from build123d import *

# Parameters (mm, degrees)
F0_R     = 1
F0_W     = 8.5
F0_H     = 8
F0_H_2   = 0.5
F1_DEPTH = 1
F2_DEPTH = 3.65
F3_DEPTH = 5.5


with BuildPart() as f1:
    # F0 (on Top) → F1 (new body)
    with BuildSketch(Plane.XY):
        Polygon((12.5, -12), (12.5, 12), (-12.5, 12), (-12.5, -12), (-10.25, -12), (-10.25, -6.25), (-4.25, -6.25), (-4.25, 1.75), (4.25, 1.75), (4.25, -6.25), (10.25, -6.25), (10.25, -12), align=None)
        with Locations((-10.5, -2.5)):
            Circle(F0_R, mode=Mode.SUBTRACT)
        with Locations((10.5, -2.5)):
            Circle(F0_R, mode=Mode.SUBTRACT)
        with Locations((-10.5, 10)):
            Circle(F0_R, mode=Mode.SUBTRACT)
        with Locations((10.5, 10)):
            Circle(F0_R, mode=Mode.SUBTRACT)
        Polygon((-10.25, -12), (10.25, -12), (10.25, -6.25), (4.25, -6.25), (4.25, -6.75), (-4.25, -6.75), (-4.25, -6.25), (-10.25, -6.25), align=None)
        with Locations((0, -2.25)):
            Rectangle(F0_W, F0_H)
        with Locations((0, -6.5)):
            Rectangle(F0_W, F0_H_2)
    extrude(amount=-F1_DEPTH)

    # F0 (on Top) → F2 (join)
    with BuildSketch(Plane.XY):
        Polygon((-10.25, -12), (10.25, -12), (10.25, -6.25), (4.25, -6.25), (4.25, -6.75), (-4.25, -6.75), (-4.25, -6.25), (-10.25, -6.25), align=None)
        with Locations((0, -6.5)):
            Rectangle(F0_W, F0_H_2)
    extrude(amount=-F2_DEPTH)

    # F0 (on Top) → F3 (join)
    with BuildSketch(Plane.XY):
        with Locations((0, -2.25)):
            Rectangle(F0_W, F0_H)
        with Locations((0, -6.5)):
            Rectangle(F0_W, F0_H_2)
    extrude(amount=F3_DEPTH)


solid = f1.part
Verification items for the finished model (mm, model axes). A direction names the side the tool comes from. Coordinates: 2 decimals unless noted, no trailing zeros. Order: outer loops, then holes, each group sorted by start corner. A loop starts at its lowest first (then second) coordinate and runs counter-clockwise, first axis right, second up. Notation, with made-up numbers: M -32.5,-35 L -2.5,-35 A8 cw -2.5,-26 Z; hole C -34,47.25 d3. An arc over 180 degrees is marked long. Write each question's results on one line, items separated by ' | '.
1) Scan lines: line 1 along Y through (x, z) = (10.5, -0.45); line 2 along Y through (x, z) = (9, -2.25); line 3 along Z through (x, y) = (-5, -1.75). Record each from-to range of solid material in increasing order. Write a range as [from, to].
Solved:
line 1: y = [-12, -3.5], [-1.5, 9], [11, 12] | line 2: y = [-12, -6.25] | line 3: z = [-1, 0]
2) Release check for a two-part mould opening along Y. For faces 4 (the face through (9.7, -3.1, -0.5)), 5 (the face through (0, -6.25, -2)), 6 (the face through (0, 3, 0)) record: pulls with the +Y half, pulls with the -Y half, needs draft (parallel to the pull), parting line crosses it, or undercut.
Solved:
face 4: undercut | face 5: pulls with the +Y half | face 6: needs draft
3) Section check D-D on x = 2. Record the cut outline in (y, z).
Solved:
outline: M -12,-3.65 L -6.25,-3.65 L -6.25,-1 L 12,-1 L 12,0 L 1.75,0 L 1.75,5.5 L -6.75,5.5 L -6.75,0 L -12,0 Z
4) Section check A-A on y = 10. Record the cut outline in (x, z), plus the area to 3 significant figures.
Solved:
outline: M -12.5,-1 L -11.5,-1 L -11.5,0 L -12.5,0 Z; M -9.5,-1 L 9.5,-1 L 9.5,0 L -9.5,0 Z; M 11.5,-1 L 12.5,-1 L 12.5,0 L 11.5,0 Z | area: 21.0 mm²
5) Gauge pin test, flat ends, axial feed: pin 1 Ø2 at (x, y) = (5.5, -2) entering from -Z; pin 2 Ø3 at (x, z) = (0, 3) entering from -Y; pin 3 Ø4.5 at (y, z) = (-1, 3.5) entering from +X; pin 4 Ø1.2 at (x, y) = (-10.5, -2.5) entering from +Z. Record the tip position at first contact, or that the pin passes through.
Solved:
pin 1: stops at z = -1 | pin 2: stops at y = -6.75 | pin 3: stops at x = 4.25 | pin 4: passes through
6) Section check B-B on z = -0.5. Record the cut outline in (x, y), plus the area to 3 significant figures.
Solved:
outline: M -12.5,-12 L 12.5,-12 L 12.5,12 L -12.5,12 Z; hole C -10.5,-2.5 d2; hole C -10.5,10 d2; hole C 10.5,-2.5 d2; hole C 10.5,10 d2 | area: 587 mm²
7) Section check C-C on y = -0.5. Record the cut outline in (x, z), plus the area to 4 significant figures.
Solved:
outline: M -12.5,-1 L 12.5,-1 L 12.5,0 L 4.25,0 L 4.25,5.5 L -4.25,5.5 L -4.25,0 L -12.5,0 Z | area: 71.75 mm²
8) Access from +Z, -Z, +X, -X, +Y, -Y to the whole of each face (thin tool, end or side, straight path). Record for faces 1 (the face through (0, 1.75, 3)), 2 (the face through (4.25, -3, 3)), 3 (the face through (-10.25, -9, -2)).
Solved:
face 1: +Z, +X, -X, +Y | face 2: +Z, +X, +Y, -Y | face 3: -Z, -X, +Y, -Y
